```python
from build123d import *

# Parameters (mm, degrees)
SKETCH1_R           = 2
SKETCH1_R_2         = 1.6000000000000019
BOSS_EXTRUDE6_DEPTH = 6
SKETCH1_6_R         = 2
BOSS_EXTRUDE7_DEPTH = 33
CUT_EXTRUDE1_START  = -12.5
CUT_EXTRUDE1_DEPTH  = 7.5
FILLET1_R           = 3
SKETCH3_R           = 1.6000000000000019
SKETCH3_R_2         = 1.6
CUT_EXTRUDE2_DEPTH  = 17.5
SKETCH4_R           = 3.4999999999999996
SKETCH4_R_2         = 1.6000000000000019
SKETCH4_R_3         = 3.5000000000000004
CUT_EXTRUDE3_DEPTH  = 3
FILLET2_R           = 3
SKETCH5_R           = 3.5
CUT_EXTRUDE6_DEPTH  = 4


with BuildPart() as part:
    # Sketch1 → Boss-Extrude6 (new body)
    # profile 1 of 2: a face of its own
    with BuildSketch(Plane.XY):
        with BuildLine():
            Line((-11.999999999999998, -8.000000000000004), (0, -8))
            ThreePointArc((0, -8), (7.9763899889711825, -0.6141683351006223), (1.2247115399099264, 7.905699314039932))
            Line((1.2247115399099258, 7.905699314039933), (-21.53439245108168, 7.905699314039933))
            ThreePointArc((-21.534392451081686, 7.90569931403993), (-20.54870521156392, 3.9952558944896794), (-20.000000000000007, -8.44e-15))
            Line((-20.000000000000004, -6.94e-15), (-19.999999999999996, -20.000000000000007))
            Line((-19.999999999999996, -20.000000000000007), (-11.999999999999998, -20.000000000000004))
            Line((-11.999999999999998, -20.000000000000004), (-11.999999999999998, -8.000000000000004))
        make_face()
        Circle(SKETCH1_R, mode=Mode.SUBTRACT)
    # profile 2 of 2: a face of its own
    with BuildSketch(Plane.XY):
        with BuildLine():
            Line((-21.53439245108168, 7.905699314039933), (1.2247115399099258, 7.905699314039933))
            ThreePointArc((1.2247115399099258, 7.905699314039921), (-11.642163108681132, 15.57150214917829), (-20.00000000000001, 28))
            ThreePointArc((-20.000000000000007, 28.000000000000004), (-33.65685424949239, 33.656854249492376), (-28.000000000000004, 20))
            ThreePointArc((-28.000000000000007, 20.000000000000004), (-24.194634546618687, 14.258940865564005), (-21.534392451081686, 7.90569931403993))
        make_face()
        with Locations((-28.000000000000007, 28.000000000000004)):
            Circle(SKETCH1_R_2, mode=Mode.SUBTRACT)
    extrude(amount=BOSS_EXTRUDE6_DEPTH)

    # Sketch1_6 → Boss-Extrude7 (add)
    with BuildSketch(Plane.XY):
        with BuildLine():
            Line((-11.999999999999998, -8.000000000000004), (0, -8))
            ThreePointArc((0, -8), (7.9763899889711825, -0.6141683351006223), (1.2247115399099264, 7.905699314039932))
            Line((1.2247115399099258, 7.905699314039933), (-21.53439245108168, 7.905699314039933))
            ThreePointArc((-21.534392451081686, 7.90569931403993), (-20.54870521156392, 3.9952558944896794), (-20.000000000000007, -8.44e-15))
            Line((-20.000000000000004, -6.94e-15), (-19.999999999999996, -20.000000000000007))
            Line((-19.999999999999996, -20.000000000000007), (-11.999999999999998, -20.000000000000004))
            Line((-11.999999999999998, -20.000000000000004), (-11.999999999999998, -8.000000000000004))
        make_face()
        Circle(SKETCH1_6_R, mode=Mode.SUBTRACT)
    extrude(amount=BOSS_EXTRUDE7_DEPTH)

    # Sketch2 → Cut-Extrude1 (cut)
    with BuildSketch(Plane.XY.offset(33).offset(CUT_EXTRUDE1_START)):
        with BuildLine():
            Line((-11.999999999999998, -8.000000000000004), (-11.999999999999998, 7.905699314039931))
            Line((-11.999999999999998, 7.905699314039931), (1.2247115399099269, 7.905699314039933))
            ThreePointArc((1.2247115399099269, 7.905699314039933), (7.976389988971184, -0.6141683351006236), (0, -8))
            Line((0, -8), (-11.999999999999998, -8.000000000000004))
        make_face()
    extrude(amount=CUT_EXTRUDE1_DEPTH, mode=Mode.SUBTRACT)

    # Fillet1
    fillet1_edges = [part.edges().sort_by_distance(p)[0] for p in [
        (-15.999999999999996, -20.000000000000007, 0),
        (-15.999999999999996, -20.000000000000007, 33),
    ]]
    fillet(fillet1_edges, radius=FILLET1_R)

    # Sketch3 → Cut-Extrude2 (cut)
    with BuildSketch(Plane(origin=(-11.999999999999998, 0, 0), x_dir=(0, 0, -1), z_dir=(1, 0, 0))):
        with Locations((-26.000000000000004, -14.000000000000004)):
            Circle(SKETCH3_R)
        with Locations((-7, -14.000000000000004)):
            Circle(SKETCH3_R_2)
    extrude(amount=-CUT_EXTRUDE2_DEPTH, mode=Mode.SUBTRACT)

    # Sketch4 → Cut-Extrude3 (cut)
    # profile 1 of 2: a face of its own
    with BuildSketch(Plane(origin=(-11.999999999999998, 0, 0), x_dir=(0, 0, -1), z_dir=(1, 0, 0))):
        with Locations((-26.000000000000004, -14.000000000000004)):
            Circle(SKETCH4_R)
        with Locations((-26.000000000000004, -14.000000000000004)):
            Circle(SKETCH4_R_2, mode=Mode.SUBTRACT)
    # profile 2 of 2: a face of its own
    with BuildSketch(Plane(origin=(-11.999999999999998, 0, 0), x_dir=(0, 0, -1), z_dir=(1, 0, 0))):
        with Locations((-7, -14.000000000000004)):
            Circle(SKETCH4_R_3)
    extrude(amount=-CUT_EXTRUDE3_DEPTH, mode=Mode.SUBTRACT)

    # Fillet2
    fillet2_edges = [part.edges().sort_by_distance(p)[0] for p in [
        (-21.534392451081686, 7.905699314039931, 19.5),
    ]]
    fillet(fillet2_edges, radius=FILLET2_R)

    # Sketch5 → Cut-Extrude6 (cut)
    with BuildSketch(Plane(origin=(0, 0, 0), x_dir=(-1, 0, 0), z_dir=(0, 0, -1))):
        Circle(SKETCH5_R)
    extrude(amount=-CUT_EXTRUDE6_DEPTH, mode=Mode.SUBTRACT)


solid = part.part
```
Can you work these out from the model? Positions are in its coordinate system, mm. A direction names the side the tool comes from. Give positions to 0.01 mm unless a question says otherwise; leave off trailing zeros. Order: outer loops, then holes, each group sorted by start corner. A loop starts at its lowest first (then second) coordinate and runs counter-clockwise, first axis right, second up. Notation, with made-up numbers: M 46,63 L 87,63 A31 ccw 87,93 Z; hole C 81.5,20 d11. An arc over 180 degrees is marked long. Write item = value, one per line. Start each with the question number.
Q1. Suppose I cut it at C-C (x = -8). Write out the boundary of the cut face in (y, z), plus the area to 3 significant figures.
Q2. Suppose I cut it at D-D (z = 26). Write out the boundary of the cut face in (x, y).
Q3. Suppose I cut it at B-B (z = 7). Write out the boundary of the cut face in (x, y), plus the area to 3 significant figures.
Q4. We'd pull the mould along Y, two halves only. Please class faces 1 (the flat face through (-15, -15, 5)), 2 (the flat face through (-16, -20, 16)), 3 (the flat face through (-4, 0, 20.5)): pulls with the +Y half, pulls with the -Y half, needs draft (parallel to the pull), parting line crosses it, or undercut.
Q5. Will these pins go through, and if not, where does the flat tip stop? pin 1 Ø1.5 at (y, z) = (6.5, 19.5) entering from +X; pin 2 Ø5.5 at (x, z) = (-8, 30.5) entering from -Y; pin 3 Ø6.5 at (x, y) = (0, 0) entering from -Z.
Q6. For faces 4 (the flat face through (-20, -10, 16)), 5 (the cylindrical face through (-13.5, -16.1, 9.8)), 6 (the flat face through (-4, 0, 28)), which set-ups out of +Z, -Z, +X, -X, +Y, -Y let a thin tool reach every point of the face, with its end or its side?
Q7. I need wall thicknesses on probe 1 along Y at (x, z) = (-17, 7); probe 2 along X at (y, z) = (0, 30); probe 3 along Y at (x, z) = (-13, 26). Which ranges of each line are inside material? Lowest first, please. Write a range as [from, to].
Q8. Suppose I cut it at A-A (y = -14). Write out the boundary of the cut face in (x, z), plus the area to 3 significant figures.
Check result:
q1.outline = M -8,0 L 12.57,0 L 12.57,6 L 7.91,6 L 7.91,20.5 L -8,20.5 Z; M -8,28 L 7.91,28 L 7.91,33 L -8,33 Z
q1.area = 434 mm2
q2.outline = M -20.61,4.31 A36.54 cw -20,0 L -20,-12.4 L -15,-12.4 L -15,-10.5 L -12,-10.5 L -12,7.91 L -17.67,7.91 A3 ccw Z; M -20,-20 L -12,-20 L -12,-17.5 L -15,-17.5 L -15,-15.6 L -20,-15.6 Z
q3.outline = M -20.61,4.31 A36.54 cw -20,0 L -20,-12.4 L -15,-12.4 L -15,-10.5 L -12,-10.5 L -12,-8 L 0,-8 A8 ccw 1.22,7.91 L -17.67,7.91 A3 ccw Z; M -20,-20 L -12,-20 L -12,-17.5 L -15,-17.5 L -15,-15.6 L -20,-15.6 Z; hole C 0,0 d4
q3.area = 467 mm2
q4.face_1 = undercut
q4.face_2 = pulls with the -Y half
q4.face_3 = needs draft
q5.pin_1 = 5.56
q5.pin_2 = -8
q5.pin_3 = 4
q6.face_4 = +Z, -Z, -X, -Y
q6.face_5 = +X
q6.face_6 = +X, +Y, -Y
q7.probe_1 = [-20, -15.6], [-12.4, 7.91]
q7.probe_2 = [-20, -2], [2, 8]
q7.probe_3 = [-20, -17.5], [-10.5, 7.91]
q8.outline = M -20,0 L -12,0 L -12,3.5 L -15,3.5 L -15,5.4 L -20,5.4 Z; M -20,8.6 L -15,8.6 L -15,10.5 L -12,10.5 L -12,22.5 L -15,22.5 L -15,24.4 L -20,24.4 Z; M -20,27.6 L -15,27.6 L -15,29.5 L -12,29.5 L -12,33 L -20,33 Z
q8.area = 190 mm2
